```python
from build123d import *

# Parameters (mm, degrees)
SKETCH_1_R               = 16.3
EXTRUDE_1_DEPTH          = 19.75
SKETCH_2_W               = 36.5
SKETCH_2_H               = 2.5
EXTRUDE_2_DEPTH          = 39.5
SKETCH_3_W               = 44.844436064
SKETCH_3_H               = 25.506740045
CUT_EXTRUDE_1_DEPTH      = 50
EXTRUDE_3_DEPTH          = 5.05
SKETCH_5_R               = 14.25
CUT_EXTRUDE_2_DEPTH      = 29.4
SKETCH_6_R               = 7.5
CUT_EXTRUDE_3_DEPTH      = 44.930797853
SKETCH_8_R               = 1.15
CUT_EXTRUDE_5_DEPTH      = 5.05
PATTERN_CIRCULAR_1_COUNT = 4
CUT_EXTRUDE_6_REACH      = 49.993
SKETCH_9_R               = 2.5
SKETCH_10_R              = 2
CUT_EXTRUDE_7_DEPTH      = 2.5
EXTRUDE_START            = -2.25
SKETCH_11_R              = 7.5
SKETCH_11_R_2            = 6.5
EXTRUDE_4_DEPTH          = 2.25
SKETCH_12_R              = 1.15
CUT_EXTRUDE_9_DEPTH      = 34.662664779
SKETCH_13_R              = 2
CUT_EXTRUDE_10_DEPTH     = 1
SKETCH_14_W              = 2.8
SKETCH_14_H              = 12
CUT_EXTRUDE_11_DEPTH     = 1.3
SKETCH_15_W              = 2.8
SKETCH_15_H              = 12
CUT_EXTRUDE_12_DEPTH     = 1.3
EXTRUDE_5_REACH          = 40.183
EXTRUDE_5_END_RADIUS     = 16.3
SKETCH_16_W              = 4
SKETCH_16_H              = 5
SKETCH_17_W              = 1
SKETCH_17_H              = 2
CUT_EXTRUDE_13_DEPTH     = 2.5
CUT_EXTRUDE_8_DEPTH      = 45.587021654
SKETCH_18_W              = 26.346157216
SKETCH_18_H              = 2.75
CUT_EXTRUDE_16_DEPTH     = 12.5
FILLET_1_R               = 2
FILLET_2_R               = 1


with BuildPart() as part:
    # 草图1 → 凸台-拉伸1 (new, symmetric)
    with BuildSketch(Plane(origin=(0, 0, 0), x_dir=(1, 0, 0), z_dir=(0, 1, 0))):
        with Locations(Location((0, 0, 0), (0, 0, 270))):
            Circle(SKETCH_1_R)
    extrude(amount=EXTRUDE_1_DEPTH, both=True)

    # 草图2 → 凸台-拉伸2 (add, through all)
    with BuildSketch(Plane.XZ.offset(19.75)):
        with Locations((3.6, -8.35)):
            Rectangle(SKETCH_2_W, SKETCH_2_H)
    extrude(amount=-EXTRUDE_2_DEPTH)

    # 草图3 → 切除-拉伸1 (cut)
    with BuildSketch(Plane.XZ.offset(19.75)):
        with Locations((-0.572218032, 5.653370022)):
            Rectangle(SKETCH_3_W, SKETCH_3_H)
    extrude(amount=-CUT_EXTRUDE_1_DEPTH, mode=Mode.SUBTRACT)

    # 草图4 → 凸台-拉伸3 (add)
    with BuildSketch(Plane.XZ.offset(19.75)):
        with BuildLine():
            Line((-14.65, -7.146152811), (-7.996542478, 4.549209646))
            ThreePointArc((-7.996542478, 4.549209646), (1.047927533, 9.140122969), (8.818653972, 2.621324497))
            ThreePointArc((8.818653972, 2.621324497), (13.721037439, -4.401937543), (21.85, -7.1))
            Line((21.85, -7.1), (-14.65, -7.146152811))
        make_face()
    extrude_3 = extrude(amount=-EXTRUDE_3_DEPTH)

    # 镜向1: 凸台-拉伸3 across plane
    add(extrude_3.mirror(Plane.ZX))

    # 草图5 → 切除-拉伸2 (cut)
    with BuildSketch(Plane(origin=(0, -14.7, 0), x_dir=(1, 0, 0), z_dir=(0, 1, 0))):
        Circle(SKETCH_5_R)
    extrude(amount=CUT_EXTRUDE_2_DEPTH, mode=Mode.SUBTRACT)

    # 草图6 → 切除-拉伸3 (cut, through all)
    with BuildSketch(Plane(origin=(0, -14.7, 0), x_dir=(1, 0, 0), z_dir=(0, 1, 0))):
        with Locations(Location((0, 0, 0), (0, 0, 270))):
            Circle(SKETCH_6_R)
    extrude(amount=-CUT_EXTRUDE_3_DEPTH, mode=Mode.SUBTRACT)

    # 草图8 → 切除-拉伸5 (cut)
    with BuildSketch(Plane(origin=(0, 19.75, 0), x_dir=(1, 0, 0), z_dir=(0, 1, 0))):
        with Locations(Location((0, -6, 0), (0, 0, 270))):
            Circle(SKETCH_8_R)
    cut_extrude_5 = extrude(amount=-CUT_EXTRUDE_5_DEPTH, mode=Mode.SUBTRACT)

    # 阵列(圆周)1: 切除-拉伸5 ×4 about axis
    pattern_circular_1_axis = Axis((0, 0, 0), (0, 1, 0))
    for i in range(1, PATTERN_CIRCULAR_1_COUNT):
        add(cut_extrude_5.rotate(pattern_circular_1_axis, i * 360 / PATTERN_CIRCULAR_1_COUNT), mode=Mode.SUBTRACT)

    # 草图9 → 切除-拉伸6 (cut, up to next)
    with BuildSketch(Plane(origin=(0, 19.75, 0), x_dir=(1, 0, 0), z_dir=(0, 1, 0)), mode=Mode.PRIVATE) as cut_extrude_6_sk1:
        with Locations(Location((0, 0, 0), (0, 0, 270))):
            Circle(SKETCH_9_R)
    cut_extrude_6_tool1 = extrude(cut_extrude_6_sk1.sketch, amount=-CUT_EXTRUDE_6_REACH, mode=Mode.PRIVATE) & part.part
    add(cut_extrude_6_tool1.solids().sort_by_distance((0, 19.75, 0))[0], mode=Mode.SUBTRACT)

    # 草图10 → 切除-拉伸7 (cut)
    with BuildSketch(Plane(origin=(0, 19.75, 0), x_dir=(1, 0, 0), z_dir=(0, 1, 0))):
        with Locations(Location((0, 6, 0), (0, 0, 270))):
            Circle(SKETCH_10_R)
        with Locations(Location((6, 0, 0), (0, 0, 270))):
            Circle(SKETCH_10_R)
        with Locations(Location((-6, 0, 0), (0, 0, 270))):
            Circle(SKETCH_10_R)
        with Locations(Location((0, -6, 0), (0, 0, 270))):
            Circle(SKETCH_10_R)
    extrude(amount=-CUT_EXTRUDE_7_DEPTH, mode=Mode.SUBTRACT)

    # 草图11 → 凸台-拉伸4 (add)
    with BuildSketch(Plane.XZ.offset(19.75).offset(EXTRUDE_START)):
        with Locations(Location((0, 0, 0), (0, 0, 90))):
            Circle(SKETCH_11_R)
        with Locations(Location((0, 0, 0), (0, 0, 270))):
            Circle(SKETCH_11_R_2, mode=Mode.SUBTRACT)
    extrude(amount=EXTRUDE_4_DEPTH)

    # 草图12 → 切除-拉伸9 (cut, through all)
    with BuildSketch(Plane.XY.offset(-7.1)):
        with Locations((17.5, 0)):
            Circle(SKETCH_12_R)
    extrude(amount=-CUT_EXTRUDE_9_DEPTH, mode=Mode.SUBTRACT)

    # 草图13 → 切除-拉伸10 (cut)
    with BuildSketch(Plane.XY.offset(-7.1)):
        with Locations((17.5, 0)):
            Circle(SKETCH_13_R)
    extrude(amount=-CUT_EXTRUDE_10_DEPTH, mode=Mode.SUBTRACT)

    # 草图14 → 切除-拉伸11 (cut)
    with BuildSketch(Plane.XY.offset(-7.1)):
        with Locations((21.85, 0)):
            Rectangle(SKETCH_14_W, SKETCH_14_H)
    extrude(amount=-CUT_EXTRUDE_11_DEPTH, mode=Mode.SUBTRACT)

    # 草图15 → 切除-拉伸12 (cut)
    with BuildSketch(Plane.XY.offset(-7.1)):
        with Locations((-14.672423113, 0)):
            Rectangle(SKETCH_15_W, SKETCH_15_H)
    extrude(amount=-CUT_EXTRUDE_12_DEPTH, mode=Mode.SUBTRACT)

    # 凸台-拉伸5: up to this cylinder (the profile starts outside it)
    extrude_5_end = Plane(origin=(0, 13.4, 0), z_dir=(0, -1, 0)) * Cylinder(EXTRUDE_5_END_RADIUS, 113.966, mode=Mode.PRIVATE)
    # 草图16 → 凸台-拉伸5 (add, up to the surface)
    with BuildSketch(Plane(origin=(0, 0, -15.1), x_dir=(-1, 0, 0), z_dir=(0, 0, -1)), mode=Mode.PRIVATE) as extrude_5_sk1:
        with Locations((11.65, 13.4)):
            Rectangle(SKETCH_16_W, SKETCH_16_H)
    extrude_5_tool1 = extrude(extrude_5_sk1.sketch, amount=-EXTRUDE_5_REACH, mode=Mode.PRIVATE) - extrude_5_end
    extrude_5 = extrude_5_tool1.solids().sort_by_distance((-11.65, 13.4, -15.1))[0]
    add(extrude_5)

    # 镜向4: 凸台-拉伸5 across plane
    add(extrude_5.mirror(Plane.ZX))

    # 草图17 → 切除-拉伸13 (cut)
    with BuildSketch(Plane(origin=(0, 0, -15.1), x_dir=(-1, 0, 0), z_dir=(0, 0, -1))):
        with Locations((11.65, 13.4)):
            Rectangle(SKETCH_17_W, SKETCH_17_H)
    cut_extrude_13 = extrude(amount=-CUT_EXTRUDE_13_DEPTH, mode=Mode.SUBTRACT)

    # 镜向5: 切除-拉伸13 across plane
    add(cut_extrude_13.mirror(Plane.ZX), mode=Mode.SUBTRACT)

    # 草图7 → 切除-拉伸8 (cut, through all)
    with BuildSketch(Plane.ZY.offset(14.65)):
        Polygon((-7.1, 19.75), (9.2, 18.323934785), (9.2, 19.75), align=None)
    cut_extrude_8 = extrude(amount=-CUT_EXTRUDE_8_DEPTH, mode=Mode.SUBTRACT)

    # 镜向3: 切除-拉伸8 across plane
    add(cut_extrude_8.mirror(Plane.ZX), mode=Mode.SUBTRACT)

    # 草图18 → 切除-拉伸16 (cut)
    with BuildSketch(Plane(origin=(0, 0, -9.6), x_dir=(-1, 0, 0), z_dir=(0, 0, -1))):
        with Locations((0, 18.375)):
            Rectangle(SKETCH_18_W, SKETCH_18_H)
    cut_extrude_16 = extrude(amount=CUT_EXTRUDE_16_DEPTH, mode=Mode.SUBTRACT)

    # 镜向6: 切除-拉伸16 across plane
    add(cut_extrude_16.mirror(Plane.ZX), mode=Mode.SUBTRACT)

    # 圆角1
    fillet_1_edges = [part.edges().sort_by_distance(p)[0] for p in [
        (12.355262037, 0, -7.1),
    ]]
    fillet(fillet_1_edges, radius=FILLET_1_R)

    # 圆角2
    fillet_2_edges = [part.edges().sort_by_distance(p)[0] for p in [
        (-12.355262037, 0, -7.1),
    ]]
    fillet(fillet_2_edges, radius=FILLET_2_R)


solid = part.part
```
Input: part model. Units: mm. Frame: model coordinates. A direction names the side the tool comes from. Coordinates: 2 decimals unless noted, no trailing zeros. Loops run counter-clockwise (first coordinate to the right, second up) from the corner with the lowest first, then second, coordinate; pieces in that order, holes last.
Q1. Line query: line 1 along Z through (x, y) = (0, 18.65); line 2 along Y through (x, z) = (17.5, -8.75); line 3 along Z through (x, y) = (-1.5, 18). Output: solid intervals per line, ascending.
Results are:
line 1: z = -9.6 to -8, -4 to -2.5, 2.5 to 4
line 2: y = -19.75 to -1.15, 1.15 to 19.75
line 3: z = -9.6 to -7.32, -4.68 to -2, 2 to 4.68, 7.32 to 9.08
Q2. Section C-C, the plane x = 6. Give the number of separate pieces and of enclosed holes in the cut face, and give its area (3 significant figures).
Results are:
separate pieces: 3
enclosed holes: 0
area: 194 mm2
Q3. Contact query for flat-ended pins moving along their axis: pin 1 (1 mm diameter, centred on y = 0.5, z = -8, fed in from -X); pin 2 (10 mm diameter, centred on x = -0.5, y = -5, fed in from +Z); pin 3 (2 mm diameter, centred on x = -11.5, y = 13.5, fed in from -Z). Output: stop coordinate, or through.
Results are:
pin 1: stops at x = -14.65
pin 2: stops at z = -13.15
pin 3: stops at z = -15.1
Q4. Mould query, pull axis Z, two halves, no side actions, for faces 4 (the flat face through (3, 19.75, -8)), 5 (the cylindrical face through (-4.85, 15.99, 0.05)), 6 (the flat face through (-11.36, 17.26, -1.36)). Classes: +Z half, -Z half, draft (parallel to the pull), parting line (faces both ways), or undercut.
Results are:
face 4: draft
face 5: undercut
face 6: +Z half
Q5. Set-up query: faces 1 (the flat face through (19, 0, -8.1)), 2 (the flat face through (-13.65, 13, -12)), 3 (the flat face through (-11.15, -13, -14)). Return all of +Z, -Z, +X, -X, +Y, -Y with unobstructed straight access to the full face (end or side cutting, diameter ignored); none if empty.
Results are:
face 1: +Z
face 2: -Z, -X, +Y, -Y
face 3: -Z
Q6. Section A-A, the plane y = 0. Return the cut outline in (x, z).
Results are:
outline: (-14.65, -9.6) - (-13.17, -9.6) arc R16.3 ccw to (13.17, -9.6) - (16.35, -9.6) - (16.35, -8.1) - (15.5, -8.1) - (15.5, -7.1) - (13.46, -7.1) arc R2 ccw to (11.81, -7.98) arc R14.25 cw to (-12.07, -7.57) arc R1 ccw to (-12.92, -7.1) - (-13.27, -7.1) - (-13.27, -8.4) - (-14.65, -8.4) - close; (18.65, -9.6) - (21.85, -9.6) - (21.85, -8.4) - (20.45, -8.4) - (20.45, -7.1) - (19.5, -7.1) - (19.5, -8.1) - (18.65, -8.1) - close
Q7. Section D-D, the plane x = 17.5. Return the cut outline in (y, z).
Results are:
outline: (-19.75, -9.6) - (-1.15, -9.6) - (-1.15, -8.1) - (-2, -8.1) - (-2, -7.1) - (-14.7, -7.1) - (-14.7, -6.39) - (-19.69, -6.39) - (-19.75, -7.1) - close; (1.15, -9.6) - (19.75, -9.6) - (19.75, -7.1) - (19.69, -6.39) - (14.7, -6.39) - (14.7, -7.1) - (2, -7.1) - (2, -8.1) - (1.15, -8.1) - close
Q8. Section B-B, the plane z = 6. Return the cut outline in (x, y), and give its area (3 significant figures).
Results are:
outline: (-6.97, -18.6) - (-2.5, -18.6) - (-2.5, -17.5) - (-4.5, -17.5) - (-4.5, -14.7) - (-6.97, -14.7) - close; (-6.97, 14.7) - (-1.15, 14.7) - (-1.15, 17.25) - (-2, 17.25) - (-2, 18.6) - (-6.97, 18.6) - close; (1.15, 14.7) - (6.97, 14.7) - (6.97, 18.6) - (2, 18.6) - (2, 17.25) - (1.15, 17.25) - close; (2.5, -18.6) - (6.97, -18.6) - (6.97, -14.7) - (4.5, -14.7) - (4.5, -17.5) - (2.5, -17.5) - close
area: 66.9 mm2
